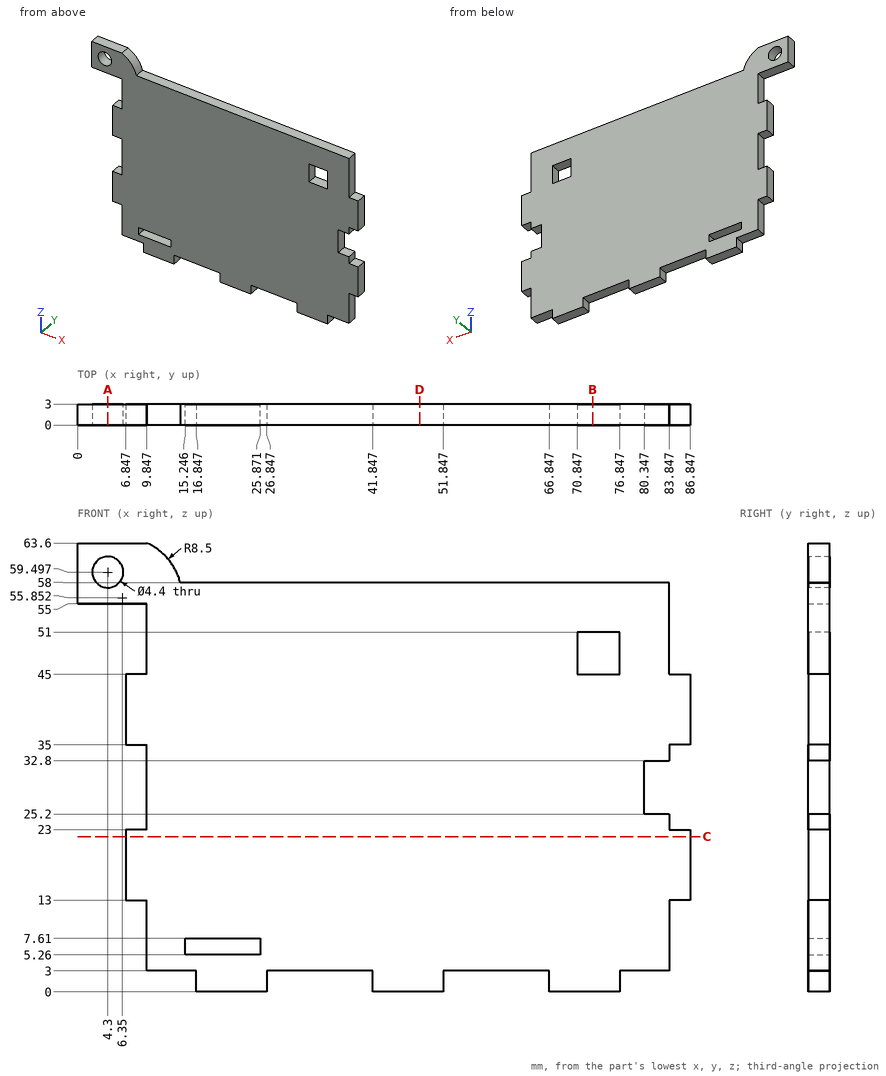
Answer from the drawing. Dimensions are ordinates in mm from the lowest x, y and z of the part. Coordinates: 2 decimals unless noted, no trailing zeros. Loops run counter-clockwise (first coordinate to the right, second up) from the corner with the lowest first, then second, coordinate; pieces in that order, holes last. Notation, with made-up numbers: (88.25, -37.5) -> (144.25, -37.5) arc R37 cw to (144.25, 1.5) -> close; hole circle Ø1 at (63.5, -10.5). An arc over 180 degrees is marked (long way). Answer in a Markdown table with one row per item.
Item 1: Each of these flat-tipped pins is pushed along its axis until it touches: P1, Ø0.9, axis at y = 1.5, z = 46.5, coming from the -X side; P2, Ø1.5, axis at y = 2, z = 2, coming from the -X side; P3, Ø1.5, axis at y = 2, z = 17, coming from the -X side. Where does it stop, or does it pass through?
Returned:
| item | result |
|---|---|
| P1 | stops at x = 9.85 |
| P2 | stops at x = 16.85 |
| P3 | stops at x = 6.85 |
Item 2: Straight lines are drawn through the part: line 1 along Z through (x, y) = (76, 1.2); line 2 along Z through (x, y) = (4.3, 1.2); line 3 along X through (y, z) = (2.95, 47). For each, find the intervals that lie inside material, in ascending order. Write a range as [from, to].
Returned:
| item | result |
|---|---|
| line 1 | z = [0, 45], [51, 58] |
| line 2 | z = [55, 57.3], [61.7, 63.6] |
| line 3 | x = [9.85, 70.85], [76.85, 83.85] |
Item 3: A cutting plane is placed at B-B on x = 73. Determine the outline of the cut face in (y, z).
Returned:
| item | result |
|---|---|
| outline | (0, 0) -> (3, 0) -> (3, 45) -> (0, 45) -> close; (0, 51) -> (3, 51) -> (3, 58) -> (0, 58) -> close |
Item 4: A cutting plane is placed at C-C on z = 22. Determine the outline of the cut face in (x, y), plus the area to 3 significant figures.
Returned:
| item | result |
|---|---|
| outline | (6.85, 0) -> (86.85, 0) -> (86.85, 3) -> (6.85, 3) -> close |
| area | 240 mm^2 |
Item 5: A cutting plane is placed at A-A on x = 4.3. Determine the outline of the cut face in (y, z), plus the area to 3 significant figures.
Returned:
| item | result |
|---|---|
| outline | (0, 55) -> (3, 55) -> (3, 57.3) -> (0, 57.3) -> close; (0, 61.7) -> (3, 61.7) -> (3, 63.6) -> (0, 63.6) -> close |
| area | 12.6 mm^2 |
Item 6: A cutting plane is placed at D-D on x = 48.5. Determine the outline of the cut face in (y, z).
Returned:
| item | result |
|---|---|
| outline | (0, 0) -> (3, 0) -> (3, 58) -> (0, 58) -> close |
